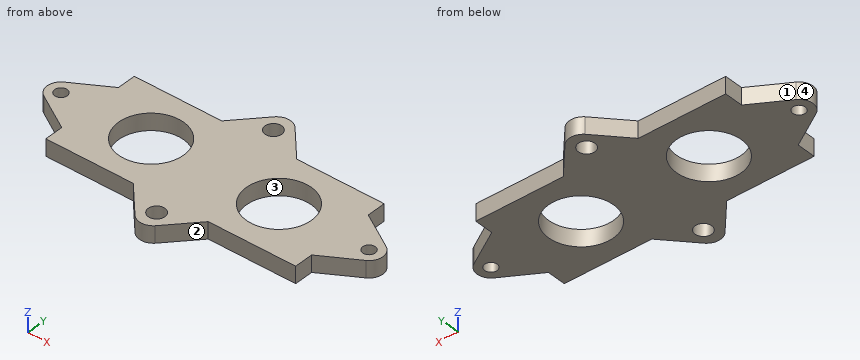
```python
from build123d import *

# Parameters (mm, degrees)
SKETCH1_R           = 7.8
SKETCH1_R_2         = 2
SKETCH1_R_3         = 1.5
BOSS_EXTRUDE1_DEPTH = 4


with BuildPart() as part:
    # Sketch1 → Boss-Extrude1 (new body)
    with BuildSketch(Plane.XY):
        with BuildLine():
            Line((-9, 12.5), (-2.401010284, 19.772380391))
            ThreePointArc((-2.401010284, 19.772380391), (0, 20.766911414), (2.401010284, 19.772380391))
            Line((2.401010284, 19.772380391), (9, 12.5))
            Line((9, 12.5), (30, 12.5))
            Line((30, 12.5), (30, 8))
            Line((30, 8), (38.682501327, 2.820305125))
            ThreePointArc((38.682501327, 2.820305125), (40.284041978, 0), (38.682501327, -2.820305125))
            Line((38.682501327, -2.820305125), (30, -8))
            Line((30, -8), (30, -12.5))
            Line((30, -12.5), (9, -12.5))
            Line((9, -12.5), (2.401010284, -19.772380391))
            ThreePointArc((2.401010284, -19.772380391), (0, -20.766911414), (-2.401010284, -19.772380391))
            Line((-2.401010284, -19.772380391), (-9, -12.5))
            Line((-9, -12.5), (-30, -12.5))
            Line((-30, -12.5), (-30, -8))
            Line((-30, -8), (-38.682501327, -2.820305125))
            ThreePointArc((-38.682501327, -2.820305125), (-40.284041978, 0), (-38.682501327, 2.820305125))
            Line((-38.682501327, 2.820305125), (-30, 8))
            Line((-30, 8), (-30, 12.5))
            Line((-30, 12.5), (-9, 12.5))
        make_face()
        with Locations((-15.35, 0)):
            Circle(SKETCH1_R, mode=Mode.SUBTRACT)
        with Locations((15.35, 0)):
            Circle(SKETCH1_R, mode=Mode.SUBTRACT)
        with Locations((0, 16.5)):
            Circle(SKETCH1_R_2, mode=Mode.SUBTRACT)
        with Locations((0, -16.5)):
            Circle(SKETCH1_R_2, mode=Mode.SUBTRACT)
        with Locations((-37, 0)):
            Circle(SKETCH1_R_3, mode=Mode.SUBTRACT)
        with Locations((37, 0)):
            Circle(SKETCH1_R_3, mode=Mode.SUBTRACT)
    extrude(amount=BOSS_EXTRUDE1_DEPTH)


solid = part.part
```
Here's how the part is built. I have some questions about the finished solid (model axes, mm). Face numbers are marked on the shaded views. Give positions to 0.01 mm unless a question says otherwise; leave off trailing zeros. Loops run counter-clockwise (first coordinate to the right, second up) from the corner with the lowest first, then second, coordinate; pieces in that order, holes last. Notation, with made-up numbers: (77.5, 57) -> (117.5, 57) arc R17 cw to (117.5, 64) -> close; hole circle Ø8 at (30.25, 1). An arc over 180 degrees is marked (long way). Use one line per item in the form item = value. Start each with the question number.
1) Thinking about a two-plate mould opening in Y: for the marked faces 1, 2, 3 and 4, which applies, +Y half, -Y half, draft (parallel to the pull), parting line (faces both ways), or undercut?
2) Imagine slicing it at D-D (x = 0). Please give me the cut outline in (y, z).
3) Imagine slicing it at A-A (y = 0). Please give me the cut outline in (x, z).
4) Imagine slicing it at C-C (z = 2.55). Please give me the cut outline in (x, y).
5) Please list where these lines run through material, in increasing order: line 1 along Y through (x, z) = (-15.35, 0.9); line 2 along X through (y, z) = (-7, 1.85); line 3 along Y through (x, z) = (-1, 3.45).
6) For P1, Ø1.8, axis at x = 37, y = 0, coming from the +Z side; P2, Ø2, axis at y = -11, z = 2, coming from the +X side; P3, Ø5, axis at x = -37, y = 0, coming from the +Z side; P4, Ø1.2, axis at y = -10, z = 2.5, coming from the -X side, each with a flat end and sliding along its axis, tell me the tip position at first contact or that it passes through.
7) Imagine slicing it at B-B (x = 15.35). Please give me the cut outline in (y, z), then the cut area to 3 significant figures.
Check values:
q1.face_1 = +Y half
q1.face_2 = -Y half
q1.face_3 = undercut
q1.face_4 = parting line
q2.outline = (-20.77, 0) -> (-18.5, 0) -> (-18.5, 4) -> (-20.77, 4) -> close; (-14.5, 0) -> (14.5, 0) -> (14.5, 4) -> (-14.5, 4) -> close; (18.5, 0) -> (20.77, 0) -> (20.77, 4) -> (18.5, 4) -> close
q3.outline = (-40.28, 0) -> (-38.5, 0) -> (-38.5, 4) -> (-40.28, 4) -> close; (-35.5, 0) -> (-23.15, 0) -> (-23.15, 4) -> (-35.5, 4) -> close; (-7.55, 0) -> (7.55, 0) -> (7.55, 4) -> (-7.55, 4) -> close; (23.15, 0) -> (35.5, 0) -> (35.5, 4) -> (23.15, 4) -> close; (38.5, 0) -> (40.28, 0) -> (40.28, 4) -> (38.5, 4) -> close
q4.outline = (-38.68, -2.82) -> (-30, -8) -> (-30, -12.5) -> (-9, -12.5) -> (-2.4, -19.77) arc R3.4 ccw to (2.4, -19.77) -> (9, -12.5) -> (30, -12.5) -> (30, -8) -> (38.68, -2.82) arc R3.28 ccw to (38.68, 2.82) -> (30, 8) -> (30, 12.5) -> (9, 12.5) -> (2.4, 19.77) arc R3.4 ccw to (-2.4, 19.77) -> (-9, 12.5) -> (-30, 12.5) -> (-30, 8) -> (-38.68, 2.82) arc R3.28 ccw to start; hole circle Ø3 at (-37, 0); hole circle Ø15.6 at (-15.35, 0); hole circle Ø4 at (0, -16.5); hole circle Ø4 at (0, 16.5); hole circle Ø15.6 at (15.35, 0); hole circle Ø3 at (37, 0)
q5.line_1 = -12.5 to -7.8, 7.8 to 12.5
q5.line_2 = -31.68 to -18.79, -11.91 to 11.91, 18.79 to 31.68
q5.line_3 = -20.62 to -18.23, -14.77 to 14.77, 18.23 to 20.62
q6.P1 = through
q6.P2 = 30
q6.P3 = 4
q6.P4 = -30
q7.outline = (-12.5, 0) -> (-7.8, 0) -> (-7.8, 4) -> (-12.5, 4) -> close; (7.8, 0) -> (12.5, 0) -> (12.5, 4) -> (7.8, 4) -> close
q7.area = 37.6 mm^2
